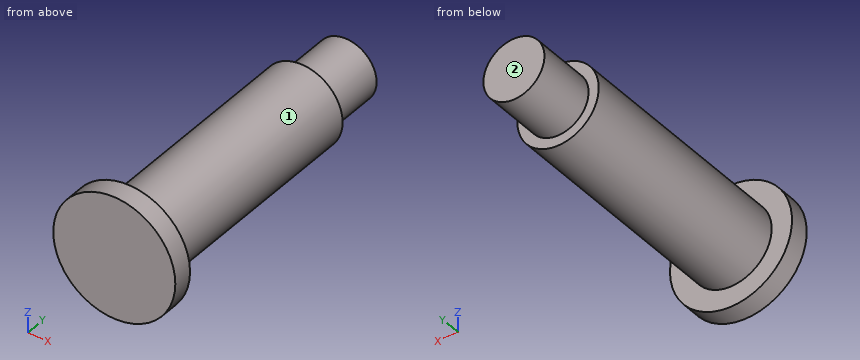
from build123d import *

# Parameters (mm, degrees)
SKETCH_1_R      = 6
EXTRUDE_1_DEPTH = 2
SKETCH_2_R      = 4
EXTRUDE_2_DEPTH = 23.5
SKETCH_3_R      = 3
EXTRUDE_3_DEPTH = 6


with BuildPart() as part:
    # 草图1 → 凸台-拉伸1 (new body)
    with BuildSketch(Plane(origin=(0, 0, 0), x_dir=(1, 0, 0), z_dir=(0, 1, 0))):
        Circle(SKETCH_1_R)
    extrude(amount=EXTRUDE_1_DEPTH)

    # 草图2 → 凸台-拉伸2 (add)
    with BuildSketch(Plane(origin=(0, 2, 0), x_dir=(1, 0, 0), z_dir=(0, 1, 0))):
        Circle(SKETCH_2_R)
    extrude(amount=EXTRUDE_2_DEPTH)

    # 草图3 → 凸台-拉伸3 (add)
    with BuildSketch(Plane(origin=(0, 25.5, 0), x_dir=(1, 0, 0), z_dir=(0, 1, 0))):
        Circle(SKETCH_3_R)
    extrude(amount=EXTRUDE_3_DEPTH)


solid = part.part
CAD build for the part. Positions are in the model's coordinates, mm. Face numbers are marked on the shaded views. A direction names the side the tool comes from. Coordinates: 2 decimals unless noted, no trailing zeros. Loops run counter-clockwise (first coordinate to the right, second up) from the corner with the lowest first, then second, coordinate; pieces in that order, holes last. Notation, with made-up numbers: (21, -33.75) - (51, -33.75) arc R12 cw to (51, -22.75) - close; hole circle Ø11 at (-32.75, -34.75). An arc over 180 degrees is marked (long way). Write item = value, one per line. Start each with the question number.
Q1. Cut at B-B, the plane x = 0. List the corners of the cut face in (y, z), then the cut area to 3 significant figures.
Q2. Cut at D-D, the plane z = -4.5. List the corners of the cut face in (x, y), then the cut area to 3 significant figures.
Q3. Cut at A-A, the plane z = 0. List the corners of the cut face in (x, y).
Q4. Drill centre lines: L1, parallel to Y at x = 4.5, z = -0.5; L2, parallel to Y at x = -0.5, z = 3; L3, parallel to Z at x = 0, y = 7. Where is each one in solid material? Low to high.
Q5. Which spindle directions (+Z, -Z, +X, -X, +Y, -Y) get a long thin tool onto all of the face, cutting with end or side? Do the marked faces 1 and 2. Say none if no direction does.
Q6. Flat gauge pins, fed straight in: pin 1 Ø5 at (y, z) = (6, 4) entering from -X; pin 2 Ø4 at (x, z) = (0, 4.5) entering from +Y; pin 3 Ø1 at (x, y) = (2, 16) entering from +Z; pin 4 Ø2 at (y, z) = (9, 0.5) entering from -X. Where does each tip first touch, or does it go through?
Q7. Cut at C-C, the plane y = 11. List the corners of the cut face in (x, z), then the cut area to 3 significant figures.
Computed:
q1.outline = (0, -6) - (2, -6) - (2, -4) - (25.5, -4) - (25.5, -3) - (31.5, -3) - (31.5, 3) - (25.5, 3) - (25.5, 4) - (2, 4) - (2, 6) - (0, 6) - close
q1.area = 248 mm²
q2.outline = (-3.97, 0) - (3.97, 0) - (3.97, 2) - (-3.97, 2) - close
q2.area = 15.9 mm²
q3.outline = (-6, 0) - (6, 0) - (6, 2) - (4, 2) - (4, 25.5) - (3, 25.5) - (3, 31.5) - (-3, 31.5) - (-3, 25.5) - (-4, 25.5) - (-4, 2) - (-6, 2) - close
q4.L1 = 0 to 2
q4.L2 = 0 to 25.5
q4.L3 = -4 to 4
q5.face_1 = +Y
q5.face_2 = +Z, -Z, +X, -X, +Y
q6.pin_1 = -3.71
q6.pin_2 = 31.5
q6.pin_3 = 3.71
q6.pin_4 = -4
q7.outline = circle Ø8 at (0, 0)
q7.area = 50.3 mm²
